from build123d import *

# Parameters (mm, degrees)
SKETCH1_R                      = 40
SKETCH1_R_2                    = 20
BOSS_EXTRUDE1_DEPTH            = 130
SKETCH2_R                      = 27.5
SKETCH2_R_2                    = 20
BOSS_EXTRUDE2_DEPTH            = 60
SKETCH2_2_R                    = 20
CUT_EXTRUDE1_DEPTH             = 61.0000001
CUT_EXTRUDE1_DEPTH_BACK        = 61.0000001
SKETCH3_R                      = 14
SKETCH3_R_2                    = 9
BOSS_EXTRUDE3_DEPTH            = 7.5
CUT_EXTRUDE2_REACH             = 132
SKETCH4_R                      = 20
CUT_EXTRUDE2_DIRECTION_2_DEPTH = 1.0000001
BOSS_EXTRUDE4_REACH            = 132
SKETCH5_R                      = 20


with BuildPart() as part:
    # Sketch1 → Boss-Extrude1 (new body)
    with BuildSketch(Plane(origin=(0, 0, 0), x_dir=(1, 0, 0), z_dir=(0, 1, 0))):
        Circle(SKETCH1_R)
        Circle(SKETCH1_R_2, mode=Mode.SUBTRACT)
    extrude(amount=BOSS_EXTRUDE1_DEPTH)

    # Sketch2 → Boss-Extrude2 (add, symmetric)
    with BuildSketch(Plane.XY):
        with Locations((0, 40)):
            Circle(SKETCH2_R)
        with Locations((0, 40)):
            Circle(SKETCH2_R_2, mode=Mode.SUBTRACT)
    extrude(amount=BOSS_EXTRUDE2_DEPTH, both=True)

    # Sketch2<2> → Cut-Extrude1 (cut, two sides)
    with BuildSketch(Plane.XY) as cut_extrude1_sk:
        with Locations((0, 40)):
            Circle(SKETCH2_2_R)
    extrude(amount=CUT_EXTRUDE1_DEPTH, mode=Mode.SUBTRACT)
    extrude(cut_extrude1_sk.sketch, amount=-CUT_EXTRUDE1_DEPTH_BACK, mode=Mode.SUBTRACT)

    # Sketch3 → Boss-Extrude3 (add, symmetric)
    with BuildSketch(Plane.XY):
        with Locations((-55, 95)):
            Circle(SKETCH3_R)
        with Locations((-55, 95)):
            Circle(SKETCH3_R_2, mode=Mode.SUBTRACT)
        with BuildLine():
            Line((-25, 111.131990931), (-40, 110.083088752))
            Line((-40, 110.083088752), (-55.976590632, 108.965896704))
            ThreePointArc((-55.976590632, 108.965896704), (-45.452022959, 105.238951823), (-41, 95))
            ThreePointArc((-41, 95), (-45.452022959, 84.761048177), (-55.976590632, 81.034103296))
            Line((-55.976590632, 81.034103296), (-40, 79.916911248))
            Line((-40, 79.916911248), (-25, 78.868009069))
            Line((-25, 78.868009069), (-25, 111.131990931))
        make_face()
        with Locations((55, 95)):
            Circle(SKETCH3_R)
        with Locations((55, 95)):
            Circle(SKETCH3_R_2, mode=Mode.SUBTRACT)
        with BuildLine():
            Line((55.976590632, 108.965896704), (40, 110.083088752))
            Line((40, 110.083088752), (25, 111.131990931))
            Line((25, 111.131990931), (25, 78.868009069))
            Line((25, 78.868009069), (40, 79.916911248))
            Line((40, 79.916911248), (55.976590632, 81.034103296))
            ThreePointArc((55.976590632, 81.034103296), (41, 95), (55.976590632, 108.965896704))
        make_face()
    extrude(amount=BOSS_EXTRUDE3_DEPTH, both=True)

    # Sketch4 → Cut-Extrude2 (cut, up to next)
    with BuildSketch(Plane(origin=(0, 130, 0), x_dir=(1, 0, 0), z_dir=(0, 1, 0)), mode=Mode.PRIVATE) as cut_extrude2_sk1:
        Circle(SKETCH4_R)
    cut_extrude2_tool1 = extrude(cut_extrude2_sk1.sketch, amount=-CUT_EXTRUDE2_REACH, mode=Mode.PRIVATE) & part.part
    add(cut_extrude2_tool1.solids().sort_by_distance((0, 130, 0))[0], mode=Mode.SUBTRACT)

    # Sketch4 → Cut-Extrude2 direction 2 (cut)
    with BuildSketch(Plane(origin=(0, 130, 0), x_dir=(1, 0, 0), z_dir=(0, 1, 0))):
        Circle(SKETCH4_R)
    extrude(amount=CUT_EXTRUDE2_DIRECTION_2_DEPTH, mode=Mode.SUBTRACT)

    # Sketch5 → Boss-Extrude4 (add, up to next)
    with BuildSketch(Plane.XZ, mode=Mode.PRIVATE) as boss_extrude4_sk1:
        Circle(SKETCH5_R)
    boss_extrude4_tool1 = extrude(boss_extrude4_sk1.sketch, amount=-BOSS_EXTRUDE4_REACH, mode=Mode.PRIVATE) - part.part
    add(boss_extrude4_tool1.solids().sort_by_distance((0, 0, 0))[0])


solid = part.part
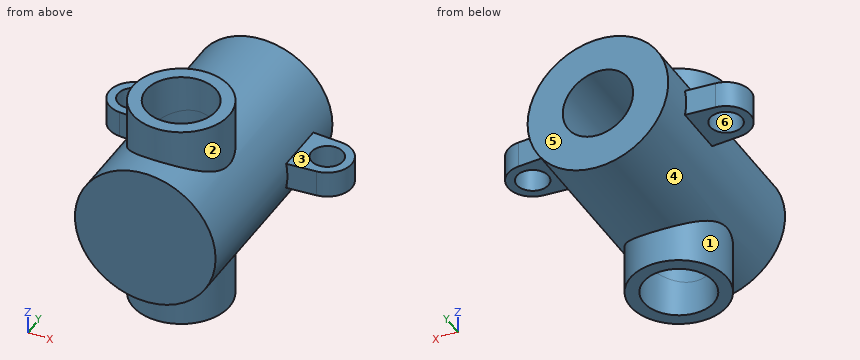
CAD build for the part. Positions are in the model's coordinates, mm. Face numbers are marked on the shaded views. A direction names the side the tool comes from. Coordinates: 2 decimals unless noted, no trailing zeros. Loops run counter-clockwise (first coordinate to the right, second up) from the corner with the lowest first, then second, coordinate; pieces in that order, holes last. Notation, with made-up numbers: (-7, 22.5) - (-2, 22.5) arc R29 cw to (-2, 45.5) - close; hole circle Ø2 at (6.5, -13). An arc over 180 degrees is marked (long way). Use one line per item in the form item = value. Start each with the question number.
1) Drill centre lines: L1, parallel to X at y = 25.5, z = -12; L2, parallel to X at y = 122.5, z = 6.5; L3, parallel to Y at x = 55, z = 4.25. Where is each one in solid material? Low to high. Write a range as from..to.
2) Two-plate mould, pull along X, no slides. Class the marked faces 4, 5 and 6: +X half, -X half, draft (parallel to the pull), parting line (faces both ways), or undercut.
3) Band-saw the part on B-B (x = 0). Give the cut face in (y, z), and give its area (3 significant figures).
4) Band-saw the part on D-D (z = 51). Give the cut face in (x, y).
5) Flat gauge pins, fed straight in: pin 1 (1.5 mm diameter, centred on x = 20.5, y = 110, fed in from -Z); pin 2 (1.5 mm diameter, centred on y = 111, z = -1, fed in from +X); pin 3 (15 mm diameter, centred on x = -61.5, y = 101, fed in from -Z); pin 4 (24 mm diameter, centred on x = 0, y = 40, fed in from +Z). Where does each tip first touch, or does it go through?
6) Tool access for the marked faces 1, 2 and 3: list every direction of +Z, -Z, +X, -X, +Y, -Y with a clear straight run to the whole face (end or side of a thin tool).
7) Band-saw the part on A-A (y = 95). Give the cut face in (x, z).
8) Band-saw the part on C-C (y = 27). Give the cut face in (x, z).
Check values:
q1.L1 = -38.16..-13.77, 13.77..38.16
q1.L2 = -39.47..-18.91, 18.91..39.47
q1.L3 = 80.97..86, 104..109.03
q2.face_4 = parting line
q2.face_5 = draft
q2.face_6 = undercut
q3.outline = (0, -40) - (12.5, -40) - (12.5, -60) - (20, -60) - (20, 60) - (12.5, 60) - (12.5, 40) - (0, 40) - close; (60, -60) - (67.5, -60) - (67.5, -40) - (130, -40) - (130, -20) - (60, -20) - close; (60, 20) - (130, 20) - (130, 40) - (67.5, 40) - (67.5, 60) - (60, 60) - close
q3.area = 5,000 mm2
q4.outline = circle Ø55 at (0, 40); hole circle Ø40 at (0, 40)
q5.pin_1 = -34.78
q5.pin_2 = 40
q5.pin_3 = -7.5
q5.pin_4 = through
q6.face_1 = -Z
q6.face_2 = +Z
q6.face_3 = +Z, +X, +Y, -Y
q7.outline = (-69, -7.5) - (-64, -7.5) - (-64, 7.5) - (-69, 7.5) - close; (-46, -7.5) - (-39.29, -7.5) arc R40 ccw to (39.29, -7.5) - (46, -7.5) - (46, 7.5) - (39.29, 7.5) arc R40 ccw to (-39.29, 7.5) - (-46, 7.5) - close; (64, -7.5) - (69, -7.5) - (69, 7.5) - (64, 7.5) - close; hole circle Ø40 at (0, 0)
q8.outline = (-24.23, -60) - (-15.2, -60) - (-15.2, 60) - (-24.23, 60) - (-24.23, 31.82) arc R40 ccw to (-24.23, -31.82) - close; (15.2, -60) - (24.23, -60) - (24.23, -31.82) arc R40 ccw to (24.23, 31.82) - (24.23, 60) - (15.2, 60) - close
